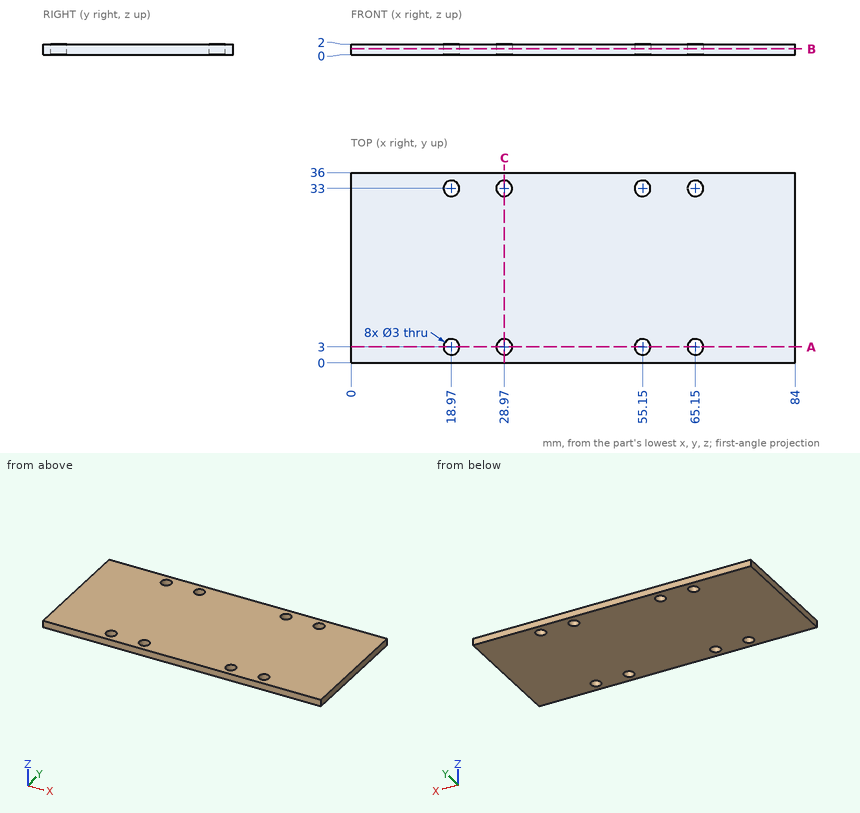
Could you check a few things on this drawing? It's one solid part, dimensions in mm from its lowest x, y, z. Round coordinates to 2 decimals unless told otherwise and drop trailing zeros. Order: outer loops, then holes, each group sorted by start corner. A loop starts at its lowest first (then second) coordinate and runs counter-clockwise, first axis right, second up. Notation, with made-up numbers: M 35.5,0.5 L 94.5,0.5 A23 cw 94.5,28.5 Z; hole C 76,25 d7. An arc over 180 degrees is marked long. Use a Markdown table: item, result.
1) Imagine slicing it at A-A (y = 3). List the corners of the cut face in (x, z) for me.
Geometry says:
| item | result |
|---|---|
| outline | M 0,0 L 17.47,0 L 17.47,2 L 0,2 Z; M 20.47,0 L 27.47,0 L 27.47,2 L 20.47,2 Z; M 30.47,0 L 53.65,0 L 53.65,2 L 30.47,2 Z; M 56.65,0 L 63.65,0 L 63.65,2 L 56.65,2 Z; M 66.65,0 L 84,0 L 84,2 L 66.65,2 Z |
2) Imagine slicing it at C-C (x = 28.97). List the corners of the cut face in (y, z) for me.
Geometry says:
| item | result |
|---|---|
| outline | M 0,0 L 1.5,0 L 1.5,2 L 0,2 Z; M 4.5,0 L 31.5,0 L 31.5,2 L 4.5,2 Z; M 34.5,0 L 36,0 L 36,2 L 34.5,2 Z |
3) I'm going to push flat-ended pins straight in: P1, Ø2.5, axis at x = 65.15, y = 33, coming from the +Z side; P2, Ø5, axis at x = 53.5, y = 28.5, coming from the -Z side. Where does each tip first touch, or does it pass through?
Geometry says:
| item | result |
|---|---|
| P1 | passes through |
| P2 | stops at z = 0 |
4) If I drill on line 1 along Y through (x, z) = (65.15, 0.85); line 2 along X through (y, z) = (33, 1.2); line 3 along X through (y, z) = (4, 0.7), over which ranges is the centre line in solid material (lowest first)?
Geometry says:
| item | result |
|---|---|
| line 1 | y = 0 to 1.5, 4.5 to 31.5, 34.5 to 36 |
| line 2 | x = 0 to 17.47, 20.47 to 27.47, 30.47 to 53.65, 56.65 to 63.65, 66.65 to 84 |
| line 3 | x = 0 to 17.85, 20.09 to 27.85, 30.09 to 54.03, 56.27 to 64.03, 66.27 to 84 |
5) Imagine slicing it at B-B (z = 1.1). Give the number of separate pieces and of enclosed holes in the cut face, then the cut area to 3 significant figures.
Geometry says:
| item | result |
|---|---|
| separate pieces | 1 |
| enclosed holes | 8 |
| area | 2,970 mm² |
